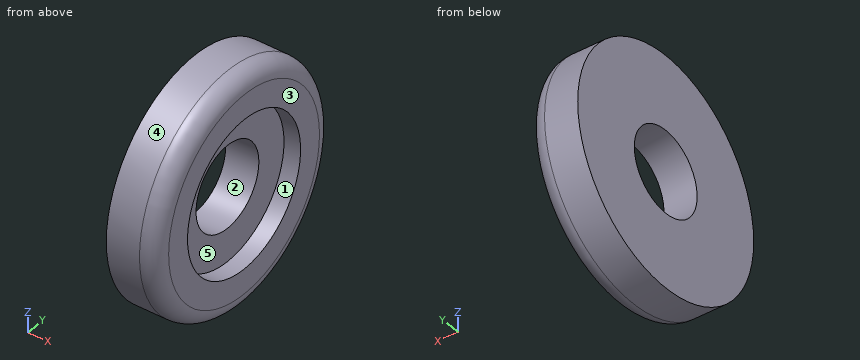
Autodesk Inventor part; units mm, degrees
ref_plane "YZ Plane" through (0, 0, 0) normal (1, 0, 0) x (0, 1, 0)
ref_plane "XZ Plane" through (0, 0, 0) normal (0, 1, 0) x (-1, 0, 0)
ref_plane "XY Plane" through (0, 0, 0) normal (0, 0, 1) x (1, 0, 0)
sketch "Sketch1" plane through (0, 0, 0) normal (1, 0, 0) x (0, 1, 0)
  circle A0 centre (0, 0) radius 3.5
  circle A1 centre (0, 0) radius 1.25
  dimension "d0" = 7
  dimension "d1" = 2.5
extrude "Extrusion1" add sketch "Sketch1" along normal blind 1.5
sketch "Sketch2" plane through (1.5, 0, 0) normal (1, 0, 0) x (0, 0, -1)
  circle A0 centre (0, 0) radius 2.25
  dimension "d4" = 4.5
extrude "Extrusion2" cut sketch "Sketch2" against normal blind 0.5
fillet "Fillet1" radius 0.5 1 edges at (1.5, -3.5, 0)
properties part number "H205_lower_linkage_washer"
Work out the finished part from the listing and answer in its coordinate system (mm). Face numbers are marked on the shaded views. A direction names the side the tool comes from. Give positions to 0.01 mm unless a question says otherwise; leave off trailing zeros. Order: outer loops, then holes, each group sorted by start corner. A loop starts at its lowest first (then second) coordinate and runs counter-clockwise, first axis right, second up.
1. The mould has two halves that part along Z. Classify the marked faces 3, 4 and 5: released by +Z, released by -Z, zero draft, split by the parting line, or undercut.
Result sheet:
face 3: zero draft
face 4: split by the parting line
face 5: undercut
2. Straight lines are drawn through the part: L1, parallel to Z at x = 0.65, y = 0; L2, parallel to Y at x = 1.3, z = 1.5; L3, parallel to Z at x = 1.35, y = -1.75. For each, find the intervals that lie inside material, in ascending order.
Result sheet:
L1: z = -3.5 to -1.25, 1.25 to 3.5
L2: y = -3.05 to -1.68, 1.68 to 3.05
L3: z = -2.86 to -1.41, 1.41 to 2.86
3. This flat-tipped pin is pushed along its axis until it touches: P1, Ø1.3, axis at y = 0.5, z = 1, coming from the +X side. Where does it stop, or does it pass through?
Result sheet:
P1: stops at x = 1
4. Section C-C, the plane x = 0.65 is taken. Determine the outline of the cut face in (y, z), and give its area (3 significant figures).
Result sheet:
outline: circle Ø7 at (0, 0); hole circle Ø2.5 at (0, 0)
area: 33.6 mm2
5. Section A-A, the plane z = 0 is taken. Determine the outline of the cut face in (x, y), and give its area (3 significant figures).
Result sheet:
outline: (0, -3.5) - (1, -3.5) arc R0.5 ccw to (1.5, -3) - (1.5, -2.25) - (1, -2.25) - (1, -1.25) - (0, -1.25) - close; (0, 1.25) - (1, 1.25) - (1, 2.25) - (1.5, 2.25) - (1.5, 3) arc R0.5 ccw to (1, 3.5) - (0, 3.5) - close
area: 5.64 mm2
6. For the marked faces 1 and 2, determine the directions among +Z, -Z, +X, -X, +Y, -Y from which every point of the face is accessible in a straight line to the end or side of a thin tool.
Result sheet:
face 1: +X
face 2: +X, -X
